Geometry check sheet. Reference: the model listing, model coordinates, mm. A direction names the side the tool comes from. Give positions to 0.01 mm unless a question says otherwise; leave off trailing zeros. Order: outer loops, then holes, each group sorted by start corner. A loop starts at its lowest first (then second) coordinate and runs counter-clockwise, first axis right, second up. Notation, with made-up numbers: M 51,54 L 103,54 A21 ccw 103,72 Z; hole C 4,61 d5. An arc over 180 degrees is marked long. One line per question, with ' | ' between items. Start each with the question number.
from build123d import *

# Parameters (mm, degrees)
F0_W     = 100
F0_H     = 100
F0_W_2   = 90
F0_H_2   = 90
F1_DEPTH = 2100
F2_R     = 20
F3_DEPTH = 100


with BuildPart() as f1:
    # F0 (on Right) → F1 (new body)
    with BuildSketch(Plane.YZ):
        Rectangle(F0_W, F0_H)
        Rectangle(F0_W_2, F0_H_2, mode=Mode.SUBTRACT)
    extrude(amount=F1_DEPTH)

    # F2 (on face) → F3 (cut)
    with BuildSketch(Plane.XZ.offset(50)):
        with Locations((1950, 0)):
            Circle(F2_R)
    extrude(amount=-F3_DEPTH, mode=Mode.SUBTRACT)


solid = f1.part
Item 1: Mould release check, pull along Z, two halves, no side actions. Record for faces 1 (the flat face through (2100, -4, -48)), 2 (the flat face through (1035, -1, -50)), 3 (the flat face through (1035, -45, -1)): released by +Z, released by -Z, zero draft, split by the parting line, or undercut.
Item 2: Cross-section at B-B, the plane z = 0. Record the cut outline in (x, y).
Item 3: Cross-section at C-C, the plane x = 1950. Record the cut outline in (y, z).
Item 4: Cross-section at A-A, the plane y = 3. Record the cut outline in (x, z).
Item 5: Cross-section at D-D, the plane x = 1072.5. Record the cut outline in (y, z).
Item 6: Material ranges on line 1 along Z through (x, y) = (267, 24.5); line 2 along Z through (x, y) = (1950, 46), recorded low to high.
Item 7: Set-up check for faces 4 (the flat face through (1035, -1, 50)), 5 (the flat face through (1035, -1, 45)): record each of +Z, -Z, +X, -X, +Y, -Y from which the full face is reachable in a straight line by a thin tool's end or side.
Outcome:
1) face 1: zero draft | face 2: released by -Z | face 3: undercut
2) outline: M 0,-50 L 1930,-50 L 1930,-45 L 0,-45 Z; M 0,45 L 1930,45 L 1930,50 L 0,50 Z; M 1970,-50 L 2100,-50 L 2100,-45 L 1970,-45 Z; M 1970,45 L 2100,45 L 2100,50 L 1970,50 Z
3) outline: M -50,-50 L 50,-50 L 50,-20 L 45,-20 L 45,-45 L -45,-45 L -45,-20 L -50,-20 Z; M -50,20 L -45,20 L -45,45 L 45,45 L 45,20 L 50,20 L 50,50 L -50,50 Z
4) outline: M 0,-50 L 2100,-50 L 2100,-45 L 0,-45 Z; M 0,45 L 2100,45 L 2100,50 L 0,50 Z
5) outline: M -50,-50 L 50,-50 L 50,50 L -50,50 Z; hole M -45,-45 L 45,-45 L 45,45 L -45,45 Z
6) line 1: z = -50 to -45, 45 to 50 | line 2: z = -50 to -20, 20 to 50
7) face 4: +Z, +X, -X, +Y, -Y | face 5: +X, -X
